Can you work these out from the drawing? Everything is in mm from the part's minimum corner. A direction names the side the tool comes from. Round coordinates to 2 decimals unless told otherwise and drop trailing zeros. Write each loop counter-clockwise with the first axis right and the second up, starting at its lowest first coordinate (ties: lowest second). Pieces come first, ordered by that corner, then holes.
Q1. If we section it at B-B (z = 56.5): Please give me the cut outline in (x, y).
Q2. If we section it at A-A (x = 3.5): Please give me the cut outline in (y, z), plus the area to 3 significant figures.
Q3. If we section it at C-C (y = 4.75): Please give me the cut outline in (x, z), plus the area to 3 significant figures.
Q4. Please list where these lines run through material, in increasing order: line 1 along X through (y, z) = (1.5, 3.5); line 2 along X through (y, z) = (19.25, 5.5).
Q5. I'm going to push flat-ended pins straight in: pin 1 Ø5.5 at (x, z) = (4, 56.5) entering from +Y; pin 2 Ø1.5 at (x, z) = (44.5, 43) entering from -Y; pin 3 Ø2 at (y, z) = (16, 4.5) entering from -X; pin 4 Ø7.5 at (x, y) = (3, 11) entering from +Z. Where does each tip first touch, or does it pass through?
Q6. For the marked faces 1, 2 and 3, which set-ups out of +Z, -Z, +X, -X, +Y, -Y let a thin tool reach every point of the face, with its end or its side?
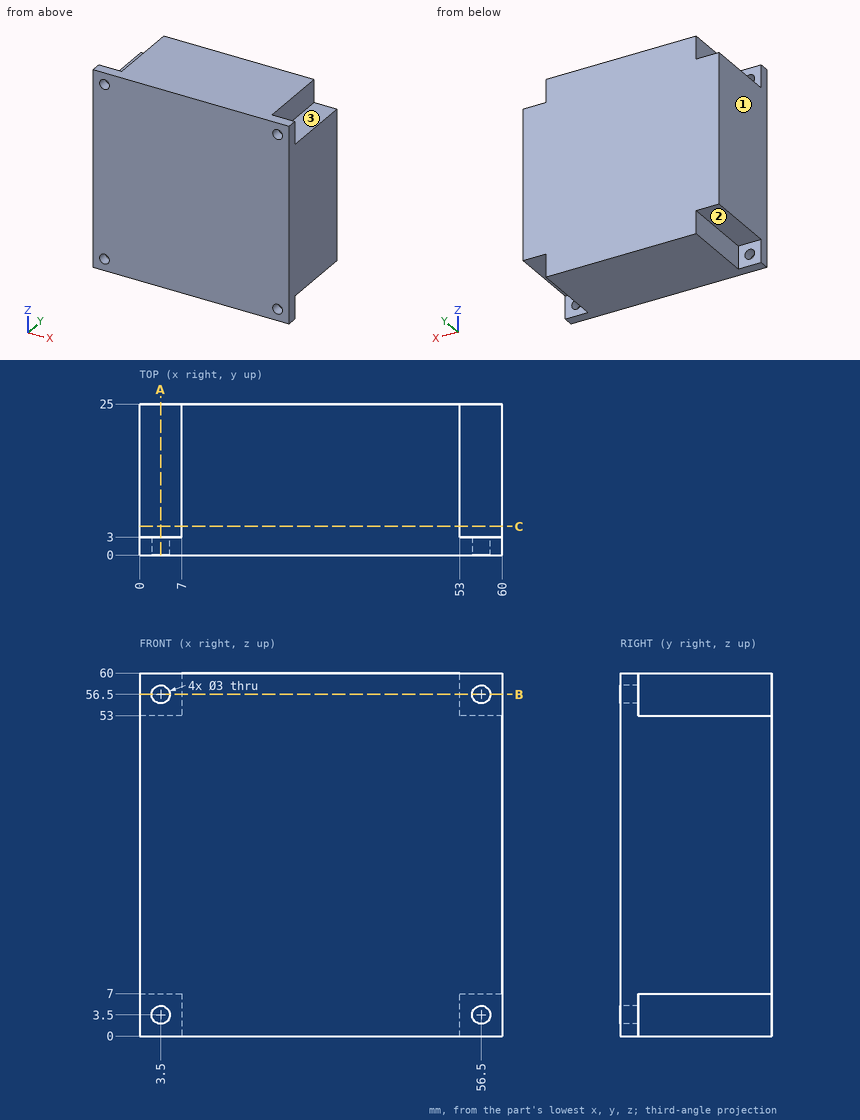
A:
1. outline: (0, 0) - (2, 0) - (2, 3) - (0, 3) - close; (5, 0) - (55, 0) - (55, 3) - (53, 3) - (53, 25) - (7, 25) - (7, 3) - (5, 3) - close; (58, 0) - (60, 0) - (60, 3) - (58, 3) - close
2. outline: (0, 0) - (3, 0) - (3, 2) - (0, 2) - close; (0, 5) - (3, 5) - (3, 7) - (25, 7) - (25, 53) - (3, 53) - (3, 55) - (0, 55) - close; (0, 58) - (3, 58) - (3, 60) - (0, 60) - close
2. area: 1,170 mm2
3. outline: (0, 7) - (7, 7) - (7, 0) - (53, 0) - (53, 7) - (60, 7) - (60, 53) - (53, 53) - (53, 60) - (7, 60) - (7, 53) - (0, 53) - close
3. area: 3,400 mm2
4. line 1: x = 0 to 2, 5 to 55, 58 to 60
4. line 2: x = 7 to 53
5. pin 1: stops at y = 3
5. pin 2: stops at y = 0
5. pin 3: stops at x = 7
5. pin 4: stops at z = 53
6. face 1: +Z, -Z, -X, +Y, -Y
6. face 2: -Z, -X, +Y
6. face 3: +Z, +X, +Y
